Drawing for the job (mm, zero at the part's lowest x, y, z). A direction names the side the tool comes from. Give positions to 0.01 mm unless a question says otherwise; leave off trailing zeros. Order: outer loops, then holes, each group sorted by start corner. A loop starts at its lowest first (then second) coordinate and runs counter-clockwise, first axis right, second up. Notation, with made-up numbers: (14, 20.25) - (63, 20.25) arc R18 ccw to (63, 37.25) - close; hole circle Ø9 at (66, 48.5). An arc over 180 degrees is marked (long way). Use a Markdown table: item, result. Add a question column.
(1) Wall check: line 1 (X direction, y = 34.5, z = 79); line 2 (Y direction, x = 8, z = 60). Give the ranges that are in metal, low to high.
(2) Slice it at C-C (x = 40.5). Write the cut outline in (y, z).
(3) Slice it at B-B (z = 29). Write the cut outline in (x, y), then the cut area to 3 significant figures.
(4) Which spindle directions (+Z, -Z, +X, -X, +Y, -Y) get a long thin tool onto all of the face, cutting with end or side? Do the marked faces 4 and 5. Say none if no direction does.
(5) Slice it at A-A (y = 7.5). Write the cut outline in (x, z), then the cut area to 3 significant figures.
(6) Flat gauge pins, fed straight in: pin 1 (5 mm diameter, centred on x = 7, y = 18.5, fed in from +Z); pin 2 (6 mm diameter, centred on x = 10.5, z = 42.5, fed in from +Y). Where does each tip first touch, or does it go through?
(7) Mould opens along X. For the marked faces 1, 2 and 3 say: +X half, -X half, draft (parallel to the pull), parting line (faces both ways), or undercut.
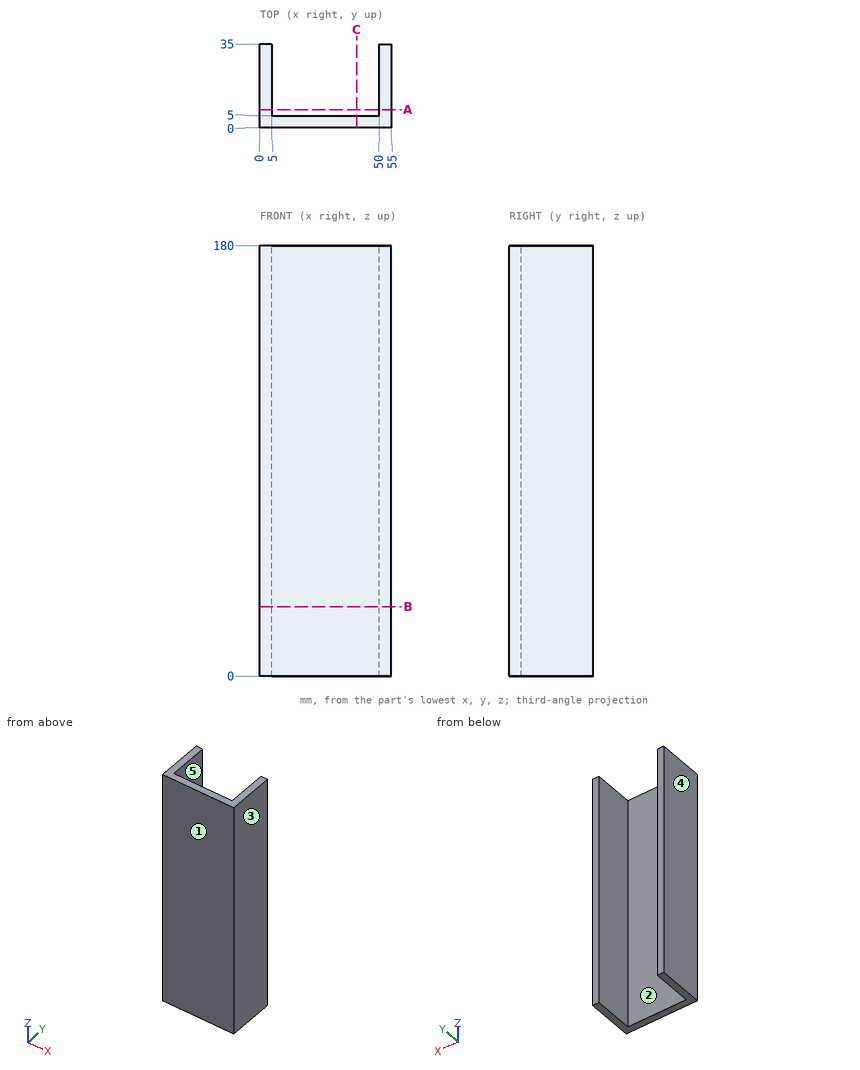
Solution:
| question | item | result |
|---|---|---|
| 1 | line 1 | 0 to 5, 50 to 55 |
| 1 | line 2 | 0 to 5 |
| 2 | outline | (0, 0) - (5, 0) - (5, 180) - (0, 180) - close |
| 3 | outline | (0, 0) - (55, 0) - (55, 35) - (50, 35) - (50, 5) - (5, 5) - (5, 35) - (0, 35) - close |
| 3 | area | 575 mm2 |
| 4 | face 4 | +Z, -Z, -X, +Y, -Y |
| 4 | face 5 | +Z, -Z, +Y |
| 5 | outline | (0, 0) - (5, 0) - (5, 180) - (0, 180) - close; (50, 0) - (55, 0) - (55, 180) - (50, 180) - close |
| 5 | area | 1,800 mm2 |
| 6 | pin 1 | z = 180 |
| 6 | pin 2 | y = 5 |
| 7 | face 1 | draft |
| 7 | face 2 | undercut |
| 7 | face 3 | +X half |
